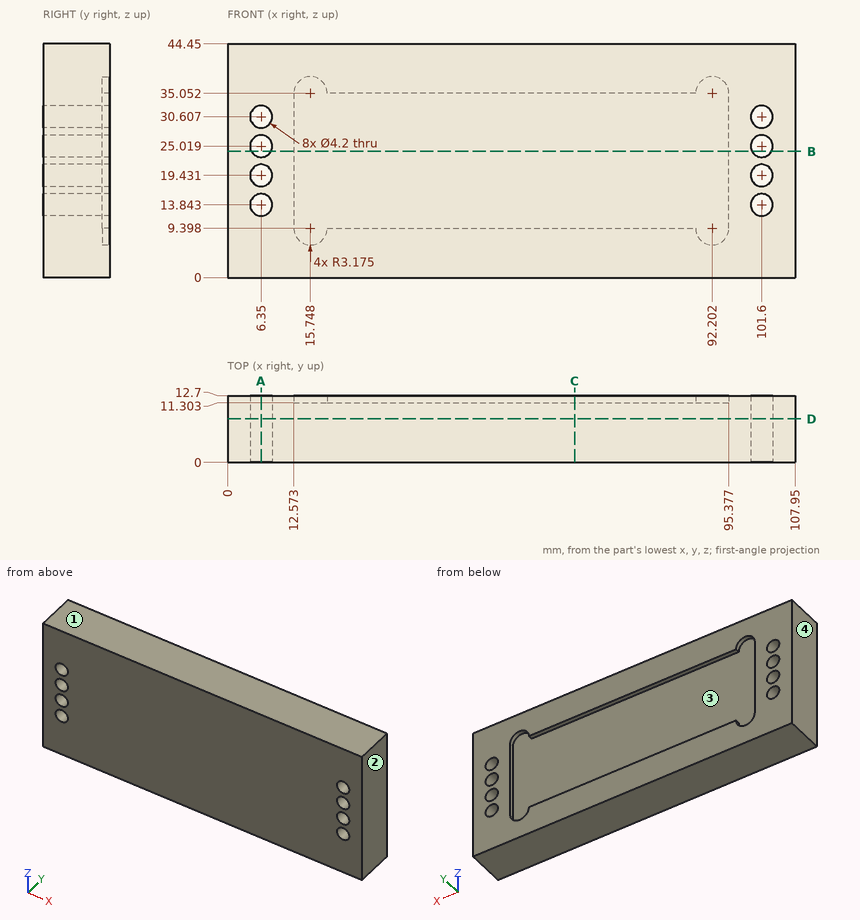
Job drawing, mm, ordinate dimensions from the low corner. One solid piece. Coordinates: 2 decimals unless noted, no trailing zeros. Order: outer loops, then holes, each group sorted by start corner. A loop starts at its lowest first (then second) coordinate and runs counter-clockwise, first axis right, second up. Notation, with made-up numbers: (84, -9) -> (100, -9) arc R19 cw to (100, 21) -> close; hole circle Ø5 at (67.5, 0). An arc over 180 degrees is marked (long way). Return JSON: item names as keys, results as strings. Group by question number.
Item 1: Saw through at C-C on x = 66. Write the cut outline in (y, z), then the cut area to 3 significant figures.
Item 2: Flat gauge pin, fed straight in: P1, Ø5, axis at x = 53, z = 14, coming from the +Y side. Where does the tip first touch, or does it go through?
Item 3: Saw through at A-A on x = 6.35. Write the cut outline in (y, z), then the cut area to 3 significant figures.
Item 4: Wall check: line 1 along Z through (x, y) = (101.6, 5); line 2 along X through (y, z) = (6.75, 32.5); line 3 along X through (y, z) = (5.5, 25.5). Give the ranges that are in metal, low to high. Write a range as [from, to].
Item 5: Saw through at B-B on z = 24. Write the cut outline in (x, y), then the cut area to 3 significant figures.
Item 6: Saw through at D-D on y = 8.25. State how many separate pieces and enclosed holes the cut face has, then the cut area to 3 significant figures.
Item 7: Pull direction X, two halves, no side cores. Call the marked faces 1, 2, 3 and 4: pulls with the +X half, pulls with the -X half, needs draft (parallel to the pull), parting line crosses it, or undercut.
Values found:
{
 "1": {"outline": "(0, 0) -> (12.7, 0) -> (12.7, 9.4) -> (11.3, 9.4) -> (11.3, 35.05) -> (12.7, 35.05) -> (12.7, 44.45) -> (0, 44.45) -> close", "area": "529 mm2"},
 "2": {"P1": "stops at y = 11.3"},
 "3": {"outline": "(0, 0) -> (12.7, 0) -> (12.7, 11.74) -> (0, 11.74) -> close; (0, 15.94) -> (12.7, 15.94) -> (12.7, 17.33) -> (0, 17.33) -> close; (0, 21.53) -> (12.7, 21.53) -> (12.7, 22.92) -> (0, 22.92) -> close; (0, 27.12) -> (12.7, 27.12) -> (12.7, 28.51) -> (0, 28.51) -> close; (0, 32.71) -> (12.7, 32.71) -> (12.7, 44.45) -> (0, 44.45) -> close", "area": "351 mm2"},
 "4": {"line 1": "z = [0, 11.74], [15.94, 17.33], [21.53, 22.92], [27.12, 28.51], [32.71, 44.45]", "line 2": "x = [0, 5.44], [7.26, 100.69], [102.51, 107.95]", "line 3": "x = [0, 4.31], [8.39, 99.56], [103.64, 107.95]"},
 "5": {"outline": "(0, 0) -> (4.51, 0) -> (4.51, 12.7) -> (0, 12.7) -> close; (8.19, 0) -> (99.76, 0) -> (99.76, 12.7) -> (95.38, 12.7) -> (95.38, 11.3) -> (12.57, 11.3) -> (12.57, 12.7) -> (8.19, 12.7) -> close; (103.44, 0) -> (107.95, 0) -> (107.95, 12.7) -> (103.44, 12.7) -> close", "area": "1,160 mm2"},
 "6": {"separate pieces": "1", "enclosed holes": "8", "area": "4,690 mm2"},
 "7": {"face 1": "needs draft", "face 2": "pulls with the +X half", "face 3": "undercut", "face 4": "pulls with the -X half"}
}
